Design review of the part built by this model. Coordinates are the model's own, in mm. Face numbers are marked on the shaded views. A direction names the side the tool comes from. Coordinates: 2 decimals unless noted, no trailing zeros. Write each loop counter-clockwise with the first axis right and the second up, starting at its lowest first coordinate (ties: lowest second). Pieces come first, ordered by that corner, then holes. Notation, with made-up numbers: (43, -40) - (99, -40) arc R18 ccw to (99, -17) - close; hole circle Ø9 at (66, 34.5). An arc over 180 degrees is marked (long way). Use a Markdown table: item, result.
from build123d import *

# Parameters (mm, degrees)
F0_R     = 5
F1_DEPTH = 10
F2_R     = 2.5
F3_DEPTH = 12.5
F0_R_2   = 7
F4_DEPTH = 0.1
F5_R     = 1
F6_R     = 0.5
F7_R     = 1
F8_DEPTH = 5


with BuildPart() as f1:
    # F0 (on Front) → F1 (new body)
    with BuildSketch(Plane.XZ):
        Circle(F0_R)
    extrude(amount=F1_DEPTH)

    # F2 (on Top) → F3 (cut, symmetric)
    with BuildSketch(Plane.XY):
        with Locations((-5, -5)):
            Circle(F2_R)
    extrude(amount=F3_DEPTH, both=True, mode=Mode.SUBTRACT)

    # F0 (on Front) → F4 (join)
    with BuildSketch(Plane.XZ):
        Circle(F0_R_2)
        Circle(F0_R, mode=Mode.SUBTRACT)
    extrude(amount=F4_DEPTH)

    # F5
    f5_edges = [f1.edges().sort_by_distance(p)[0] for p in [
        (-5, -0.1, 0),
        (-5, -10, 0),
    ]]
    fillet(f5_edges, radius=F5_R)

    # F6
    f6_edges = [f1.edges().sort_by_distance(p)[0] for p in [
        (5, -5.05, 0),
        (-5, -1.1, 0),
        (-5, -9, 0),
        (-2.5, -5, 4.330127),
    ]]
    fillet(f6_edges, radius=F6_R)

    # F7 (on Front) → F8 (cut)
    with BuildSketch(Plane.XZ):
        Circle(F7_R)
    extrude(amount=F8_DEPTH, mode=Mode.SUBTRACT)


solid = f1.part
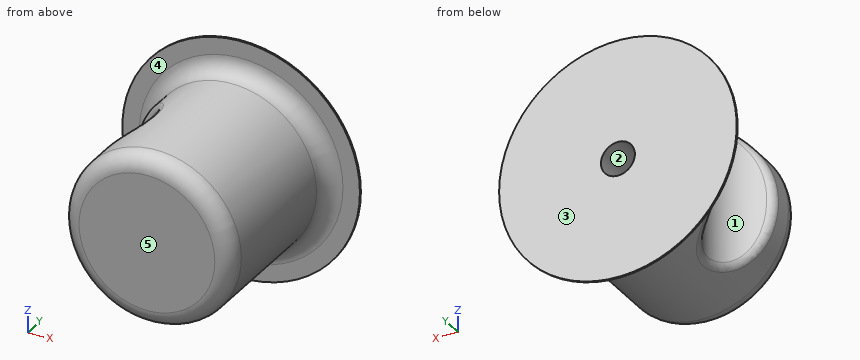
(1) For pin 1 (2 mm diameter, centred on x = 2, y = -4, fed in from -Z); pin 2 (6 mm diameter, centred on x = 1.5, y = -4, fed in from -Z); pin 3 (4 mm diameter, centred on x = 4, y = -7.5, fed in from -Z), all flat-tipped, find the tip position at first contact; note any pin that passes through.
Determined:
| item | result |
|---|---|
| pin 1 | z = -4.9 |
| pin 2 | z = -5 |
| pin 3 | z = -4.58 |
(2) Draft analysis for pull direction Y (two halves, no side actions). For the marked faces 1, 2 and 3, state which applies: +Y half, -Y half, draft (parallel to the pull), parting line (faces both ways), or undercut.
Determined:
| item | result |
|---|---|
| face 1 | undercut |
| face 2 | draft |
| face 3 | +Y half |
(3) Take a section at A-A on y = -0.5. Write out the cut boundary in (x, z).
Determined:
| item | result |
|---|---|
| outline | circle Ø10.4 at (0, 0); hole circle Ø2 at (0, 0) |
(4) For L1, parallel to Z at x = 0, y = -3.1; L2, parallel to Y at x = -3.5, z = 0.75; L3, parallel to Y at x = 0.75, z = 0, list the stretches that pass through material, from the lowest coordinate up. Write a range as from..to.
Determined:
| item | result |
|---|---|
| L1 | -5..-1, 1..5 |
| L2 | -10..-7, -3..0 |
| L3 | -10..-5 |
(5) Machinability: for the marked faces 4 and 5, which of the approach directions +Z, -Z, +X, -X, +Y, -Y give a long, thin tool a straight path to every point of the face, cutting with its end or side? Answer none if there is none.
Determined:
| item | result |
|---|---|
| face 4 | -Y |
| face 5 | +Z, -Z, +X, -X, -Y |
(6) Take a section at B-B on x = 0. Write out the cut boundary in (y, z).
Determined:
| item | result |
|---|---|
| outline | (-10, -4) arc R1 ccw to (-9, -5) - (-1.1, -5) arc R1 cw to (-0.1, -6) - (-0.1, -7) - (0, -7) - (0, -1) - (-5, -1) - (-5, 1) - (0, 1) - (0, 7) - (-0.1, 7) - (-0.1, 6) arc R1 cw to (-1.1, 5) - (-9, 5) arc R1 ccw to (-10, 4) - close |
